Verification items for this drawing (mm, ordinates from the low corner). A direction names the side the tool comes from. Round coordinates to 2 decimals unless told otherwise and drop trailing zeros. Order: outer loops, then holes, each group sorted by start corner. A loop starts at its lowest first (then second) coordinate and runs counter-clockwise, first axis right, second up. Notation, with made-up numbers: (15.5, 65) - (64.5, 65) arc R17 ccw to (64.5, 75) - close; hole circle Ø1 at (0.25, -9). An arc over 180 degrees is marked (long way). One line per question, with ' | ' between items. Start each with the question number.
Q1. Sectioned sample at A-A, the plane y = 21.11. Enter the section's corners in (x, z) (1 decimal), then the cut area to 3 significant figures.
Q2. Sectioned sample at C-C, the plane z = 14. Enter the section's corners in (x, y) (1 decimal).
Q3. Material ranges on line 1 along Z through (x, y) = (5.5, 27); line 2 along X through (y, z) = (24, 14) (1 decimal); line 3 along Y through (x, z) = (3.25, 14.25) (1 decimal), recorded low to high.
Q4. Sectioned sample at B-B, the plane x = 6. Enter the section's corners in (y, z) (1 decimal).
Q5. Sectioned sample at D-D, the plane x = 1. Enter the section's corners in (y, z), then the cut area to 3 significant figures.
Q6. Tool access check on the marked faces 1 and 2. Record the directions out of +Z, -Z, +X, -X, +Y, -Y that give a thin tool (end or side, any length) a straight path to the whole face; none if there is none.
Q7. Gauge pin test, flat end, axial feed: P1, Ø1, axis at x = 6.5, y = 10, coming from the +Z side. Record the tip position at first contact, or that the pin passes through.
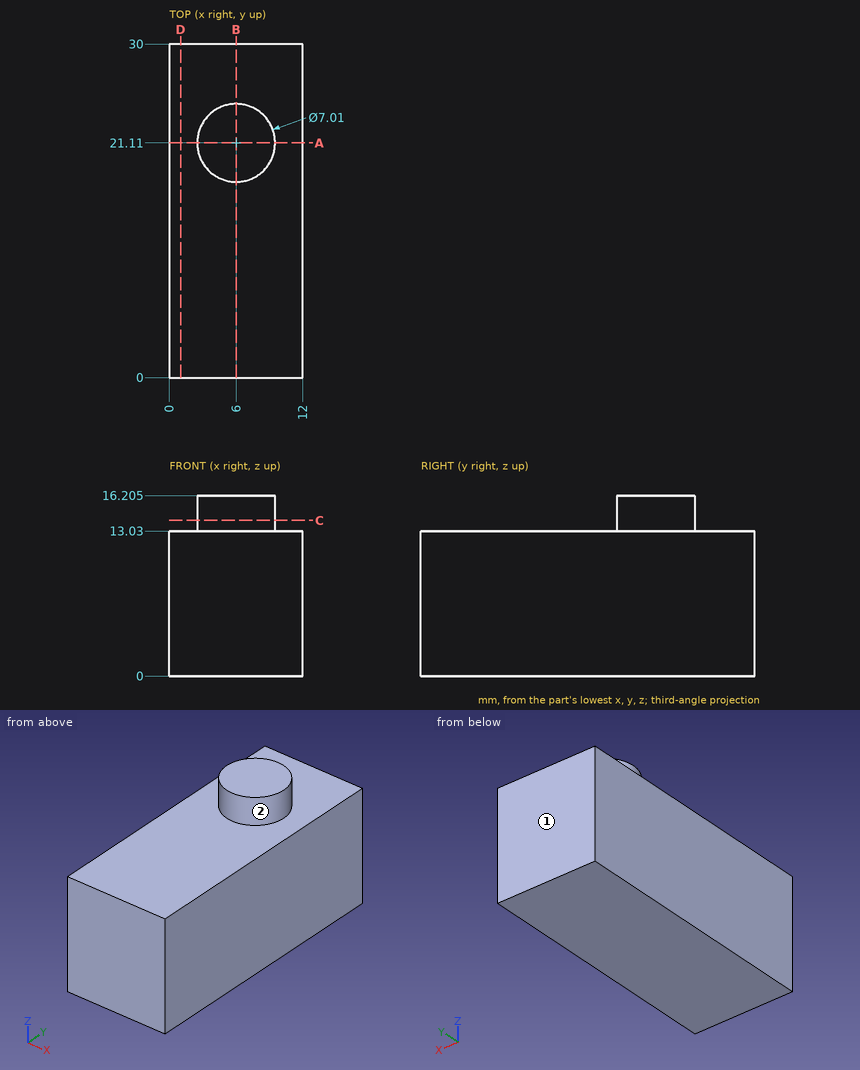
Determined:
1) outline: (0, 0) - (12, 0) - (12, 13) - (9.5, 13) - (9.5, 16.2) - (2.5, 16.2) - (2.5, 13) - (0, 13) - close | area: 179 mm2
2) outline: circle Ø7 at (6, 21.1)
3) line 1: z = 0 to 13.03 | line 2: x = 4 to 8 | line 3: y = 18.9 to 23.3
4) outline: (0, 0) - (30, 0) - (30, 13) - (24.6, 13) - (24.6, 16.2) - (17.6, 16.2) - (17.6, 13) - (0, 13) - close
5) outline: (0, 0) - (30, 0) - (30, 13.03) - (0, 13.03) - close | area: 391 mm2
6) face 1: +Z, -Z, +X, -X, +Y | face 2: +Z
7) P1: stops at z = 13.03
